The drawing under review shows one solid part. Ordinate dimensions are in mm from its lowest x, y, z. Round coordinates to 2 decimals unless told otherwise and drop trailing zeros. Write each loop counter-clockwise with the first axis right and the second up, starting at its lowest first coordinate (ties: lowest second). Pieces come first, ordered by that corner, then holes.
Item 1: Add section A-A (x = 170.5). Give the boundary of the cut face in (y, z).
Item 2: To check wall thickness, follow L1, parallel to Y at x = 155, z = 5.25; L2, parallel to X at y = 32, z = 1.5; L3, parallel to Y at x = 105, z = 6.5. State the ranges of each line that lie inside material, in increasing order.
Item 3: Clearance check with flat-ended pins moving along their axes: pin 1 Ø1.5 at (x, z) = (1.5, 5) entering from -Y; pin 2 Ø5 at (y, z) = (43, 3.5) entering from -X. State where each tip first meets the part, or that it passes through.
Item 4: Add section B-B (y = 43). Give the boundary of the cut face in (x, z).
Item 5: Add section D-D (y = 17.5). Give the boundary of the cut face in (x, z).
Item 6: Add section C-C (z = 5.25). Give the boundary of the cut face in (x, y).
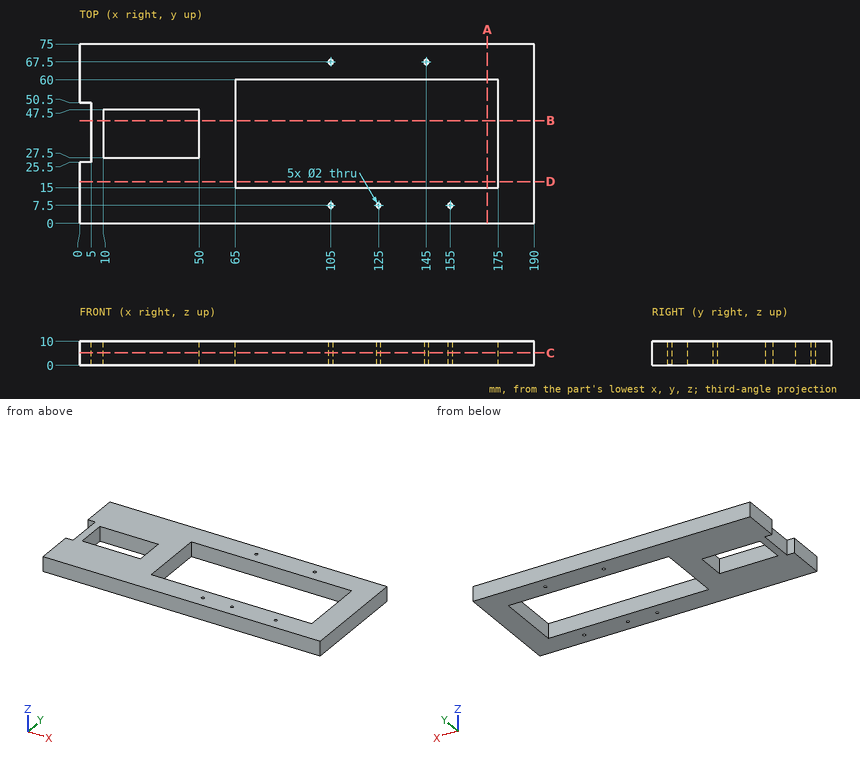
Numbers:
1. outline: (0, 0) - (15, 0) - (15, 10) - (0, 10) - close; (60, 0) - (75, 0) - (75, 10) - (60, 10) - close
2. L1: y = 0 to 6.5, 8.5 to 15, 60 to 75
2. L2: x = 5 to 10, 50 to 65, 175 to 190
2. L3: y = 0 to 6.5, 8.5 to 15, 60 to 66.5, 68.5 to 75
3. pin 1: stops at y = 0
3. pin 2: stops at x = 5
4. outline: (5, 0) - (10, 0) - (10, 10) - (5, 10) - close; (50, 0) - (65, 0) - (65, 10) - (50, 10) - close; (175, 0) - (190, 0) - (190, 10) - (175, 10) - close
5. outline: (0, 0) - (65, 0) - (65, 10) - (0, 10) - close; (175, 0) - (190, 0) - (190, 10) - (175, 10) - close
6. outline: (0, 0) - (190, 0) - (190, 75) - (0, 75) - (0, 50.5) - (5, 50.5) - (5, 25.5) - (0, 25.5) - close; hole (10, 27.5) - (50, 27.5) - (50, 47.5) - (10, 47.5) - close; hole (65, 15) - (175, 15) - (175, 60) - (65, 60) - close; hole circle Ø2 at (105, 7.5); hole circle Ø2 at (105, 67.5); hole circle Ø2 at (125, 7.5); hole circle Ø2 at (145, 67.5); hole circle Ø2 at (155, 7.5)
